```python
from build123d import *

# Parameters (mm, degrees)
SKETCH_1_W           = 250
SKETCH_1_H           = 150
EXTRUDE_1_DEPTH      = 5
SKETCH_1_4_R         = 3
CUT_EXTRUDE_1_DEPTH  = 5
SKETCH_1_5_R         = 3
CUT_EXTRUDE_2_DEPTH  = 5
SKETCH_1_6_R         = 3
CUT_EXTRUDE_3_DEPTH  = 5
SKETCH_1_7_R         = 3
CUT_EXTRUDE_4_DEPTH  = 5
SKETCH_2_R           = 3
CUT_EXTRUDE_5_DEPTH  = 5
SKETCH_3_R           = 3
CUT_EXTRUDE_6_DEPTH  = 45
SKETCH_3_3_R         = 3.5
CUT_EXTRUDE_7_DEPTH  = 45
SKETCH_4_R           = 3
CUT_EXTRUDE_8_DEPTH  = 5
SKETCH_4_3_R         = 3
CUT_EXTRUDE_9_DEPTH  = 5
SKETCH_5_R           = 3
CUT_EXTRUDE_10_DEPTH = 5
SKETCH_6_W           = 250
SKETCH_6_H           = 150
SKETCH_6_R           = 3
SKETCH_6_R_2         = 3.5
CUT_EXTRUDE_11_DEPTH = 1.5
SKETCH_7_R           = 3
CUT_EXTRUDE_12_DEPTH = 205.296965225


with BuildPart() as part:
    # Sketch 1 → Extrude 1 (new body)
    with BuildSketch(Plane(origin=(0, 0, 0), x_dir=(1, 0, 0), z_dir=(0, 1, 0))):
        with Locations((-65, 0)):
            Rectangle(SKETCH_1_W, SKETCH_1_H)
    extrude(amount=-EXTRUDE_1_DEPTH)

    # Sketch 1_4 → Cut-Extrude 1 (cut)
    with BuildSketch(Plane(origin=(0, 0, 0), x_dir=(1, 0, 0), z_dir=(0, 1, 0))):
        with Locations(Location((0, 50, 0), (0, 0, 270))):
            Circle(SKETCH_1_4_R)
    extrude(amount=-CUT_EXTRUDE_1_DEPTH, mode=Mode.SUBTRACT)

    # Sketch 1_5 → Cut-Extrude 2 (cut)
    with BuildSketch(Plane(origin=(0, 0, 0), x_dir=(1, 0, 0), z_dir=(0, 1, 0))):
        with Locations(Location((-50, 0, 0), (0, 0, 270))):
            Circle(SKETCH_1_5_R)
    extrude(amount=-CUT_EXTRUDE_2_DEPTH, mode=Mode.SUBTRACT)

    # Sketch 1_6 → Cut-Extrude 3 (cut)
    with BuildSketch(Plane(origin=(0, 0, 0), x_dir=(1, 0, 0), z_dir=(0, 1, 0))):
        with Locations(Location((0, -50, 0), (0, 0, 270))):
            Circle(SKETCH_1_6_R)
    extrude(amount=-CUT_EXTRUDE_3_DEPTH, mode=Mode.SUBTRACT)

    # Sketch 1_7 → Cut-Extrude 4 (cut)
    with BuildSketch(Plane(origin=(0, 0, 0), x_dir=(1, 0, 0), z_dir=(0, 1, 0))):
        with Locations(Location((50, 0, 0), (0, 0, 270))):
            Circle(SKETCH_1_7_R)
    extrude(amount=-CUT_EXTRUDE_4_DEPTH, mode=Mode.SUBTRACT)

    # Sketch 2 → Cut-Extrude 5 (cut)
    with BuildSketch(Plane(origin=(0, 0, 0), x_dir=(1, 0, 0), z_dir=(0, 1, 0))):
        with Locations(Location((-170.76, -37.46, 0), (0, 0, 270))):
            Circle(SKETCH_2_R)
    extrude(amount=-CUT_EXTRUDE_5_DEPTH, mode=Mode.SUBTRACT)

    # Sketch 3 → Cut-Extrude 6 (cut)
    with BuildSketch(Plane(origin=(0, 0, 0), x_dir=(1, 0, 0), z_dir=(0, 1, 0))):
        with Locations(Location((-152.57, -37.93, 0), (0, 0, 270))):
            Circle(SKETCH_3_R)
    extrude(amount=-CUT_EXTRUDE_6_DEPTH, mode=Mode.SUBTRACT)

    # Sketch 3_3 → Cut-Extrude 7 (cut)
    with BuildSketch(Plane(origin=(0, 0, 0), x_dir=(1, 0, 0), z_dir=(0, 1, 0))):
        with Locations(Location((-158.16, -24.34, 0), (0, 0, 270))):
            Circle(SKETCH_3_3_R)
    extrude(amount=-CUT_EXTRUDE_7_DEPTH, mode=Mode.SUBTRACT)

    # Sketch 4 → Cut-Extrude 8 (cut)
    with BuildSketch(Plane(origin=(0, 0, 0), x_dir=(1, 0, 0), z_dir=(0, 1, 0))):
        with Locations(Location((-112.5, -50, 0), (0, 0, 270))):
            Circle(SKETCH_4_R)
    extrude(amount=-CUT_EXTRUDE_8_DEPTH, mode=Mode.SUBTRACT)

    # Sketch 4_3 → Cut-Extrude 9 (cut)
    with BuildSketch(Plane(origin=(0, 0, 0), x_dir=(1, 0, 0), z_dir=(0, 1, 0))):
        with Locations(Location((-64.5, -50, 0), (0, 0, 270))):
            Circle(SKETCH_4_3_R)
    extrude(amount=-CUT_EXTRUDE_9_DEPTH, mode=Mode.SUBTRACT)

    # Sketch 5 → Cut-Extrude 10 (cut)
    with BuildSketch(Plane(origin=(0, 0, 0), x_dir=(1, 0, 0), z_dir=(0, 1, 0))):
        with Locations(Location((-132.61, -18.84, 0), (0, 0, 270))):
            Circle(SKETCH_5_R)
        with Locations(Location((-121.14, 21.42, 0), (0, 0, 270))):
            Circle(SKETCH_5_R)
    extrude(amount=-CUT_EXTRUDE_10_DEPTH, mode=Mode.SUBTRACT)

    # Sketch 6 → Cut-Extrude 11 (cut)
    with BuildSketch(Plane(origin=(0, 0, 0), x_dir=(1, 0, 0), z_dir=(0, 1, 0))):
        with Locations((-65, 0)):
            Rectangle(SKETCH_6_W, SKETCH_6_H)
        with Locations(Location((-170.76, -37.46, 0), (0, 0, 270))):
            Circle(SKETCH_6_R, mode=Mode.SUBTRACT)
        with Locations(Location((-158.16, -24.34, 0), (0, 0, 270))):
            Circle(SKETCH_6_R_2, mode=Mode.SUBTRACT)
        with Locations(Location((-152.57, -37.93, 0), (0, 0, 270))):
            Circle(SKETCH_6_R, mode=Mode.SUBTRACT)
        with Locations(Location((-132.61, -18.84, 0), (0, 0, 270))):
            Circle(SKETCH_6_R, mode=Mode.SUBTRACT)
        with Locations(Location((-112.5, -50, 0), (0, 0, 270))):
            Circle(SKETCH_6_R, mode=Mode.SUBTRACT)
        with Locations(Location((-121.14, 21.42, 0), (0, 0, 270))):
            Circle(SKETCH_6_R, mode=Mode.SUBTRACT)
        with Locations(Location((-50, 0, 0), (0, 0, 270))):
            Circle(SKETCH_6_R, mode=Mode.SUBTRACT)
        with Locations(Location((-64.5, -50, 0), (0, 0, 270))):
            Circle(SKETCH_6_R, mode=Mode.SUBTRACT)
        with Locations(Location((0, 50, 0), (0, 0, 270))):
            Circle(SKETCH_6_R, mode=Mode.SUBTRACT)
        with Locations(Location((0, -50, 0), (0, 0, 270))):
            Circle(SKETCH_6_R, mode=Mode.SUBTRACT)
        with Locations(Location((50, 0, 0), (0, 0, 270))):
            Circle(SKETCH_6_R, mode=Mode.SUBTRACT)
    extrude(amount=-CUT_EXTRUDE_11_DEPTH, mode=Mode.SUBTRACT)

    # Sketch 7 → Cut-Extrude 12 (cut, through all)
    with BuildSketch(Plane(origin=(0, -1.5, 0), x_dir=(1, 0, 0), z_dir=(0, 1, 0))):
        with Locations(Location((-64.5, 50, 0), (0, 0, 270))):
            Circle(SKETCH_7_R)
        with Locations(Location((-112.5, 50, 0), (0, 0, 270))):
            Circle(SKETCH_7_R)
        with Locations(Location((-64.5, -50, 0), (0, 0, 270))):
            Circle(SKETCH_7_R)
        with Locations(Location((-112.5, -50, 0), (0, 0, 270))):
            Circle(SKETCH_7_R)
    extrude(amount=-CUT_EXTRUDE_12_DEPTH, mode=Mode.SUBTRACT)


solid = part.part
```
For this review, take the finished solid that the model builds, in its own axes (mm). Give positions to 0.01 mm unless a question says otherwise; leave off trailing zeros. Write each loop counter-clockwise with the first axis right and the second up, starting at its lowest first coordinate (ties: lowest second). Pieces come first, ordered by that corner, then holes.
Item 1: Take a section at B-B (x = -121.14). Give the boundary of the cut face in (y, z), and give its area (3 significant figures).
Item 2: Take a section at A-A (z = 0). Give the boundary of the cut face in (x, y), and give its area (3 significant figures).
Item 3: Take a section at D-D (z = 50). Give the boundary of the cut face in (x, y), and give its area (3 significant figures).
Item 4: Insertion check: P1, Ø9.5, axis at x = -50, z = 0, coming from the +Y side. The pin has a flat end and moves straight along its axis. Give the tip position at first contact, or say it passes through.
Item 5: Take a section at C-C (z = 24.34). Give the boundary of the cut face in (x, y), and give its area (4 significant figures).
Item 6: The part is to be moulded in two halves that separate along X. For faces 1 (the face through (-130.08, -3.23, 20.45)), 2 (the face through (-67, -5, -1)), say which applies: +X half, -X half, draft (parallel to the pull), parting line (faces both ways), or undercut.
Item 7: Wall thickness on probe 1 along X at (y, z) = (-3.6, -50); probe 2 along X at (y, z) = (-3.9, 37.46); probe 3 along Z at (x, y) = (-170.76, -2.4): over which ranges is each line inside the solid? List them lowest first.
Established:
1. outline: (-5, -75) - (-1.5, -75) - (-1.5, -24.42) - (-5, -24.42) - close; (-5, -18.42) - (-1.5, -18.42) - (-1.5, 75) - (-5, 75) - close
1. area: 504 mm2
2. outline: (-190, -5) - (-53, -5) - (-53, -1.5) - (-190, -1.5) - close; (-47, -5) - (47, -5) - (47, -1.5) - (-47, -1.5) - close; (53, -5) - (60, -5) - (60, -1.5) - (53, -1.5) - close
2. area: 833 mm2
3. outline: (-190, -5) - (-115.5, -5) - (-115.5, -1.5) - (-190, -1.5) - close; (-109.5, -5) - (-67.5, -5) - (-67.5, -1.5) - (-109.5, -1.5) - close; (-61.5, -5) - (-3, -5) - (-3, -1.5) - (-61.5, -1.5) - close; (3, -5) - (60, -5) - (60, -1.5) - (3, -1.5) - close
3. area: 812 mm2
4. P1: stops at y = -1.5
5. outline: (-190, -5) - (-161.66, -5) - (-161.66, -1.5) - (-190, -1.5) - close; (-154.66, -5) - (60, -5) - (60, -1.5) - (-154.66, -1.5) - close
5. area: 850.5 mm2
6. face 1: undercut
6. face 2: draft
7. probe 1: x = -190 to -115.5, -109.5 to -67.5, -61.5 to -3, 3 to 60
7. probe 2: x = -190 to -173.76, -167.76 to -155.53, -149.61 to 60
7. probe 3: z = -75 to 34.46, 40.46 to 75
